The drawing under review shows one solid part. Ordinate dimensions are in mm from its lowest x, y, z. Round coordinates to 2 decimals unless told otherwise and drop trailing zeros. Write each loop counter-clockwise with the first axis right and the second up, starting at its lowest first coordinate (ties: lowest second). Pieces come first, ordered by that corner, then holes. Notation, with made-up numbers: M 28.25,55.5 L 57.25,55.5 A26 cw 57.25,73.5 Z; hole C 35,14.5 d4. An arc over 180 degrees is marked long. One line per item, written item: value. Start each with the question number.
1) For P1, Ø8, axis at x = 70, z = 47, coming from the -Y side; P2, Ø5.5, axis at x = 27.54, z = 19.12, coming from the -Y side, all flat-tipped, find the tip position at first contact; note any pin that passes through.
2) Wall thickness on probe 1 along Z at (x, y) = (32, 3.2) (1 decimal); probe 2 along Z at (x, y) = (33.5, 4.35); probe 3 along X at (y, z) = (3.45, 7.5) (1 decimal): over which ranges is each line inside the solid? List them lowest first.
3) Take a section at B-B, the plane y = 3.75. State how many separate pieces and enclosed holes the cut face has, and give its area (3 significant figures).
4) Take a section at C-C, the plane z = 62. Write out the cut boundary in (x, y) (1 decimal), and give its area (3 significant figures).
5) Take a section at A-A, the plane x = 72. Write out the cut boundary in (y, z) (1 decimal), and give its area (3 significant figures).
6) Take a section at D-D, the plane x = 86.5. Write out the cut boundary in (y, z) (1 decimal).
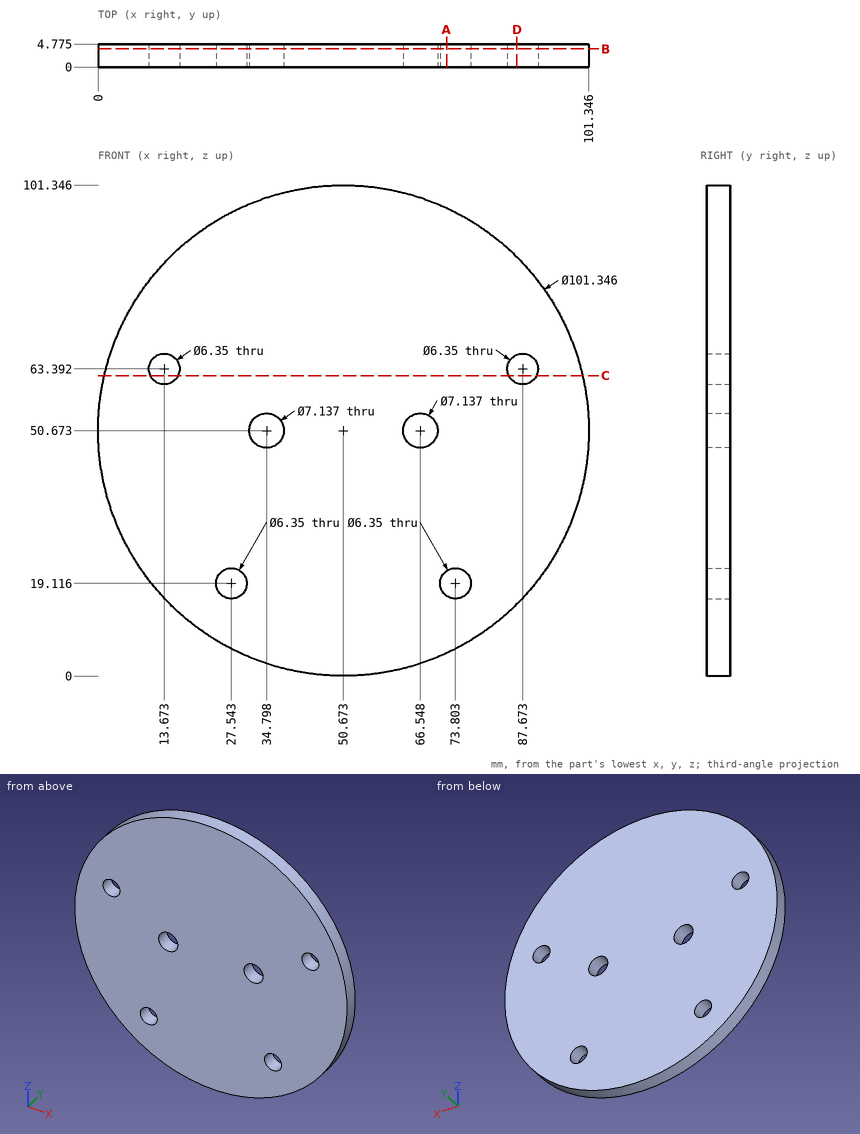
Checked values:
1. P1: stops at y = 0
1. P2: passes through
2. probe 1: z = 3.6 to 48.5, 52.9 to 97.8
2. probe 2: z = 3 to 47.35, 54 to 98.35
2. probe 3: x = 24.1 to 77.2
3. separate pieces: 1
3. enclosed holes: 6
3. area: 7,860 mm2
4. outline: M 1.3,0 L 10.8,0 L 10.8,4.8 L 1.3,4.8 Z; M 16.5,0 L 84.8,0 L 84.8,4.8 L 16.5,4.8 Z; M 90.5,0 L 100.1,0 L 100.1,4.8 L 90.5,4.8 Z
4. area: 417 mm2
5. outline: M 0,4.7 L 4.8,4.7 L 4.8,16.5 L 0,16.5 Z; M 0,21.7 L 4.8,21.7 L 4.8,96.6 L 0,96.6 Z
5. area: 414 mm2
6. outline: M 0,14.8 L 4.8,14.8 L 4.8,60.4 L 0,60.4 Z; M 0,66.3 L 4.8,66.3 L 4.8,86.5 L 0,86.5 Z
